```python
from build123d import *

# Parameters (mm, degrees)
SKETCH1_W           = 40
SKETCH1_H           = 40
BOSS_EXTRUDE1_DEPTH = 1.5
SKETCH2_W           = 40
SKETCH2_H           = 1.5
BOSS_EXTRUDE2_DEPTH = 45.5
CUT_EXTRUDE2_REACH  = 75.546
CUT_EXTRUDE3_REACH  = 75.546
SKETCH4_R           = 1.7
CUT_EXTRUDE4_REACH  = 74.596
SKETCH5_R           = 1.8
FILLET1_R           = 2


with BuildPart() as part:
    # Sketch1 → Boss-Extrude1 (new body)
    with BuildSketch(Plane(origin=(0, 0, 0), x_dir=(1, 0, 0), z_dir=(0, 1, 0))):
        with Locations((20, 20)):
            Rectangle(SKETCH1_W, SKETCH1_H)
    extrude(amount=BOSS_EXTRUDE1_DEPTH)

    # Sketch2 → Boss-Extrude2 (add)
    with BuildSketch(Plane(origin=(0, 1.5, 0), x_dir=(1, 0, 0), z_dir=(0, 1, 0))):
        with Locations((20, 39.25)):
            Rectangle(SKETCH2_W, SKETCH2_H)
    extrude(amount=BOSS_EXTRUDE2_DEPTH)

    # Sketch3 → Cut-Extrude2 (cut, up to next)
    with BuildSketch(Plane(origin=(0, 0, -40), x_dir=(-1, 0, 0), z_dir=(0, 0, -1)), mode=Mode.PRIVATE) as cut_extrude2_sk1:
        with BuildLine():
            Line((-13.5, 20), (-13.5, 34))
            ThreePointArc((-13.5, 34), (-20, 40.5), (-26.5, 34))
            Line((-26.5, 34), (-26.5, 20))
            ThreePointArc((-26.5, 20), (-20, 13.5), (-13.5, 20))
        make_face()
    cut_extrude2_tool1 = extrude(cut_extrude2_sk1.sketch, amount=-CUT_EXTRUDE2_REACH, mode=Mode.PRIVATE) & part.part
    # Sketch3 → Cut-Extrude2 (cut, up to next)
    with BuildSketch(Plane(origin=(0, 0, -40), x_dir=(-1, 0, 0), z_dir=(0, 0, -1)), mode=Mode.PRIVATE) as cut_extrude2_sk2:
        with BuildLine():
            Line((-20, 47), (-40, 47))
            Line((-40, 47), (-40, 27))
            ThreePointArc((-40, 27), (-34.142135624, 41.142135624), (-20, 47))
        make_face()
    cut_extrude2_tool2 = extrude(cut_extrude2_sk2.sketch, amount=-CUT_EXTRUDE2_REACH, mode=Mode.PRIVATE) & part.part
    # Sketch3 → Cut-Extrude2 (cut, up to next)
    with BuildSketch(Plane(origin=(0, 0, -40), x_dir=(-1, 0, 0), z_dir=(0, 0, -1)), mode=Mode.PRIVATE) as cut_extrude2_sk3:
        with BuildLine():
            Line((0, 47), (-20, 47))
            ThreePointArc((-20, 47), (-5.857864376, 41.142135624), (0, 27))
            Line((0, 27), (0, 47))
        make_face()
    cut_extrude2_tool3 = extrude(cut_extrude2_sk3.sketch, amount=-CUT_EXTRUDE2_REACH, mode=Mode.PRIVATE) & part.part
    add(cut_extrude2_tool1.solids().sort_by_distance((20, 27, -40))[0], mode=Mode.SUBTRACT)
    add(cut_extrude2_tool2.solids().sort_by_distance((35.532641, 42.532641, -40))[0], mode=Mode.SUBTRACT)
    add(cut_extrude2_tool3.solids().sort_by_distance((4.467359, 42.532641, -40))[0], mode=Mode.SUBTRACT)

    # Sketch4 → Cut-Extrude3 (cut, up to next)
    with BuildSketch(Plane(origin=(0, 0, -40), x_dir=(-1, 0, 0), z_dir=(0, 0, -1)), mode=Mode.PRIVATE) as cut_extrude3_sk1:
        with Locations((-35.5, 27)):
            Circle(SKETCH4_R)
    cut_extrude3_tool1 = extrude(cut_extrude3_sk1.sketch, amount=-CUT_EXTRUDE3_REACH, mode=Mode.PRIVATE) & part.part
    # Sketch4 → Cut-Extrude3 (cut, up to next)
    with BuildSketch(Plane(origin=(0, 0, -40), x_dir=(-1, 0, 0), z_dir=(0, 0, -1)), mode=Mode.PRIVATE) as cut_extrude3_sk2:
        with Locations((-27.75, 40.423393759)):
            Circle(SKETCH4_R)
    cut_extrude3_tool2 = extrude(cut_extrude3_sk2.sketch, amount=-CUT_EXTRUDE3_REACH, mode=Mode.PRIVATE) & part.part
    # Sketch4 → Cut-Extrude3 (cut, up to next)
    with BuildSketch(Plane(origin=(0, 0, -40), x_dir=(-1, 0, 0), z_dir=(0, 0, -1)), mode=Mode.PRIVATE) as cut_extrude3_sk3:
        with Locations((-12.25, 40.423393759)):
            Circle(SKETCH4_R)
    cut_extrude3_tool3 = extrude(cut_extrude3_sk3.sketch, amount=-CUT_EXTRUDE3_REACH, mode=Mode.PRIVATE) & part.part
    # Sketch4 → Cut-Extrude3 (cut, up to next)
    with BuildSketch(Plane(origin=(0, 0, -40), x_dir=(-1, 0, 0), z_dir=(0, 0, -1)), mode=Mode.PRIVATE) as cut_extrude3_sk4:
        with Locations((-4.5, 27)):
            Circle(SKETCH4_R)
    cut_extrude3_tool4 = extrude(cut_extrude3_sk4.sketch, amount=-CUT_EXTRUDE3_REACH, mode=Mode.PRIVATE) & part.part
    # Sketch4 → Cut-Extrude3 (cut, up to next)
    with BuildSketch(Plane(origin=(0, 0, -40), x_dir=(-1, 0, 0), z_dir=(0, 0, -1)), mode=Mode.PRIVATE) as cut_extrude3_sk5:
        with Locations((-12.25, 13.576606241)):
            Circle(SKETCH4_R)
    cut_extrude3_tool5 = extrude(cut_extrude3_sk5.sketch, amount=-CUT_EXTRUDE3_REACH, mode=Mode.PRIVATE) & part.part
    # Sketch4 → Cut-Extrude3 (cut, up to next)
    with BuildSketch(Plane(origin=(0, 0, -40), x_dir=(-1, 0, 0), z_dir=(0, 0, -1)), mode=Mode.PRIVATE) as cut_extrude3_sk6:
        with Locations((-27.75, 13.576606241)):
            Circle(SKETCH4_R)
    cut_extrude3_tool6 = extrude(cut_extrude3_sk6.sketch, amount=-CUT_EXTRUDE3_REACH, mode=Mode.PRIVATE) & part.part
    add(cut_extrude3_tool1.solids().sort_by_distance((35.5, 27, -40))[0], mode=Mode.SUBTRACT)
    add(cut_extrude3_tool2.solids().sort_by_distance((27.75, 40.423394, -40))[0], mode=Mode.SUBTRACT)
    add(cut_extrude3_tool3.solids().sort_by_distance((12.25, 40.423394, -40))[0], mode=Mode.SUBTRACT)
    add(cut_extrude3_tool4.solids().sort_by_distance((4.5, 27, -40))[0], mode=Mode.SUBTRACT)
    add(cut_extrude3_tool5.solids().sort_by_distance((12.25, 13.576606, -40))[0], mode=Mode.SUBTRACT)
    add(cut_extrude3_tool6.solids().sort_by_distance((27.75, 13.576606, -40))[0], mode=Mode.SUBTRACT)

    # Sketch5 → Cut-Extrude4 (cut, up to next)
    with BuildSketch(Plane(origin=(0, 1.5, 0), x_dir=(1, 0, 0), z_dir=(0, 1, 0)), mode=Mode.PRIVATE) as cut_extrude4_sk1:
        with Locations(Location((5, 32, 0), (0, 0, 270))):
            Circle(SKETCH5_R)
    cut_extrude4_tool1 = extrude(cut_extrude4_sk1.sketch, amount=-CUT_EXTRUDE4_REACH, mode=Mode.PRIVATE) & part.part
    # Sketch5 → Cut-Extrude4 (cut, up to next)
    with BuildSketch(Plane(origin=(0, 1.5, 0), x_dir=(1, 0, 0), z_dir=(0, 1, 0)), mode=Mode.PRIVATE) as cut_extrude4_sk2:
        with Locations(Location((35, 32, 0), (0, 0, 270))):
            Circle(SKETCH5_R)
    cut_extrude4_tool2 = extrude(cut_extrude4_sk2.sketch, amount=-CUT_EXTRUDE4_REACH, mode=Mode.PRIVATE) & part.part
    # Sketch5 → Cut-Extrude4 (cut, up to next)
    with BuildSketch(Plane(origin=(0, 1.5, 0), x_dir=(1, 0, 0), z_dir=(0, 1, 0)), mode=Mode.PRIVATE) as cut_extrude4_sk3:
        with Locations(Location((35, 8, 0), (0, 0, 270))):
            Circle(SKETCH5_R)
    cut_extrude4_tool3 = extrude(cut_extrude4_sk3.sketch, amount=-CUT_EXTRUDE4_REACH, mode=Mode.PRIVATE) & part.part
    # Sketch5 → Cut-Extrude4 (cut, up to next)
    with BuildSketch(Plane(origin=(0, 1.5, 0), x_dir=(1, 0, 0), z_dir=(0, 1, 0)), mode=Mode.PRIVATE) as cut_extrude4_sk4:
        with Locations(Location((5, 8, 0), (0, 0, 270))):
            Circle(SKETCH5_R)
    cut_extrude4_tool4 = extrude(cut_extrude4_sk4.sketch, amount=-CUT_EXTRUDE4_REACH, mode=Mode.PRIVATE) & part.part
    add(cut_extrude4_tool1.solids().sort_by_distance((5, 1.5, -32))[0], mode=Mode.SUBTRACT)
    add(cut_extrude4_tool2.solids().sort_by_distance((35, 1.5, -32))[0], mode=Mode.SUBTRACT)
    add(cut_extrude4_tool3.solids().sort_by_distance((35, 1.5, -8))[0], mode=Mode.SUBTRACT)
    add(cut_extrude4_tool4.solids().sort_by_distance((5, 1.5, -8))[0], mode=Mode.SUBTRACT)

    # Fillet1
    fillet1_edges = [part.edges().sort_by_distance(p)[0] for p in [
        (20, 1.5, -38.5),
        (20, 0, -40),
        (40, 0.75, 0),
        (0, 0.75, 0),
    ]]
    fillet(fillet1_edges, radius=FILLET1_R)


solid = part.part
```
The model under review builds one solid part; all positions refer to its coordinate system, in mm. A direction names the side the tool comes from. Round coordinates to 2 decimals unless told otherwise and drop trailing zeros. Order: outer loops, then holes, each group sorted by start corner. A loop starts at its lowest first (then second) coordinate and runs counter-clockwise, first axis right, second up. Notation, with made-up numbers: (-16, 1) -> (26, 1) arc R19 ccw to (26, 8) -> close; hole circle Ø5 at (-22, 39.25). An arc over 180 degrees is marked (long way). One line per item, written item: value. Start each with the question number.
Q1. Machinability: for faces 1 (the face through (3.905, 0.76, -9.428)), 2 (the face through (20.1, 13.5, -39.3)), 3 (the face through (15, 15, -38.5)), which of the approach directions +Z, -Z, +X, -X, +Y, -Y give a long, thin tool a straight path to every point of the face, cutting with its end or side? Answer none if there is none.
Q2. Wall thickness on line 1 (X direction, y = 0.45, z = -8); line 2 (Y direction, x = 27, z = -39) (3 decimals); line 3 (Z direction, x = 35, y = 6): over which ranges is each line inside the solid? List them lowest first.
Q3. Clearance check with flat-ended pins moving along their axes: pin 1 Ø4 at (x, z) = (5, -32) entering from -Y; pin 2 Ø11 at (x, z) = (24.5, -23.5) entering from +Y; pin 3 Ø2 at (x, z) = (5, -8) entering from -Y; pin 4 Ø4 at (x, y) = (27.75, 13.58) entering from +Z. State where each tip first meets the part, or that it passes through.
Q4. Take a section at A-A (z = -32). Write out the cut boundary in (x, y), and give its area (3 significant figures).
Q5. Take a section at B-B (x = 5). Write out the cut boundary in (y, z).
Q6. Take a section at D-D (y = 37). Write out the cut boundary in (x, z), and give its area (3 significant figures).
Q7. Mouldability with a two-part tool opening along Z and no side actions: class faces 4 (the face through (40, 1, -27)), 5 (the face through (15, 14, -40)), 6 (the face through (36.785, 0.76, -8.234)) as released by +Z, released by -Z, zero draft, split by the parting line, or undercut.
Q8. Take a section at C-C (x = 27.75). Write out the cut boundary in (y, z).
Reported:
1. face 1: +Y, -Y
1. face 2: +Z, -Z
1. face 3: +Z, +X, -X, +Y
2. line 1: x = 0 to 3.2, 6.8 to 33.2, 36.8 to 40
2. line 2: y = 0.268 to 12.051, 15.102 to 38.898, 41.949 to 45.735
2. line 3: z = -40 to -38.5
3. pin 1: stops at y = 0
3. pin 2: stops at y = 1.5
3. pin 3: passes through
3. pin 4: stops at z = -38.5
4. outline: (0, 0) -> (3.2, 0) -> (3.2, 1.5) -> (0, 1.5) -> close; (6.8, 0) -> (33.2, 0) -> (33.2, 1.5) -> (6.8, 1.5) -> close; (36.8, 0) -> (40, 0) -> (40, 1.5) -> (36.8, 1.5) -> close
4. area: 49.2 mm2
5. outline: (0, -38) arc R2 ccw to (2, -40) -> (25.38, -40) -> (25.38, -38.5) -> (3.5, -38.5) arc R2 cw to (1.5, -36.5) -> (1.5, -33.8) -> (0, -33.8) -> close; (0, -30.2) -> (1.5, -30.2) -> (1.5, -9.8) -> (0, -9.8) -> close; (0, -6.2) -> (1.5, -6.2) -> (1.5, 0) -> (0, 0) -> close; (28.62, -40) -> (40.23, -40) -> (40.23, -38.5) -> (28.62, -38.5) -> close
6. outline: (2.68, -40) -> (14.23, -40) -> (14.23, -38.5) -> (2.68, -38.5) -> close; (25.77, -40) -> (37.32, -40) -> (37.32, -38.5) -> (25.77, -38.5) -> close
6. area: 34.7 mm2
7. face 4: zero draft
7. face 5: released by -Z
7. face 6: undercut
8. outline: (0, -38) arc R2 ccw to (2, -40) -> (11.88, -40) -> (11.88, -38.5) -> (3.5, -38.5) arc R2 cw to (1.5, -36.5) -> (1.5, 0) -> (0, 0) -> close; (15.28, -40) -> (38.72, -40) -> (38.72, -38.5) -> (15.28, -38.5) -> close; (42.12, -40) -> (45.44, -40) -> (45.44, -38.5) -> (42.12, -38.5) -> close
